Check sheet for the modelled part. Datum: model origin and axes. Units: mm. A direction names the side the tool comes from. Coordinates: 2 decimals unless noted, no trailing zeros. Loops run counter-clockwise (first coordinate to the right, second up) from the corner with the lowest first, then second, coordinate; pieces in that order, holes last. Notation, with made-up numbers: (73, 16) -> (90, 16) arc R16 ccw to (90, 25) -> close; hole circle Ø3 at (-1.75, 37). An arc over 180 degrees is marked (long way). Use one line per item in the form item = value.
from build123d import *

# Parameters (mm, degrees)
SKETCH2_R           = 3
BOSS_EXTRUDE1_DEPTH = 1


with BuildPart() as part:
    # Sketch1 → Revolve1 (revolve)
    with BuildSketch(Plane.XY, mode=Mode.PRIVATE) as revolve1_sk:
        Polygon((0, 0), (2.5, 0), (2.5, 4), (7.5, 4), (7.5, 6), (10, 6), (10, 4), (12.497669608, 4), (12.497669608, 14), (10, 14), (10, 12), (7.5, 12), (7.5, 14), (5, 14), (5, 29), (0, 29), align=None)
    revolve(revolve1_sk.sketch.rotate(Axis((0, 0, 0), (0, 1, 0)), 90), axis=Axis((0, 0, 0), (0, 1, 0)))

    # Sketch2 → Boss-Extrude1 (add)
    with BuildSketch(Plane.XZ.offset(-4)):
        with Locations(Location((0, 0, 0), (0, 0, 270))):
            Circle(SKETCH2_R)
    extrude(amount=BOSS_EXTRUDE1_DEPTH)


solid = part.part
(1) Section check C-C, the plane z = 6.25. Record the boundary of the cut face in (x, y).
Established:
outline = (-10.82, 4) -> (-7.81, 4) -> (-7.81, 6) -> (-4.15, 6) -> (-4.15, 4) -> (4.15, 4) -> (4.15, 6) -> (7.81, 6) -> (7.81, 4) -> (10.82, 4) -> (10.82, 14) -> (7.81, 14) -> (7.81, 12) -> (4.15, 12) -> (4.15, 14) -> (-4.15, 14) -> (-4.15, 12) -> (-7.81, 12) -> (-7.81, 14) -> (-10.82, 14) -> close
(2) Scan lines: line 1 along X through (y, z) = (5.45, 0); line 2 along Y through (x, z) = (-10.75, 0.75); line 3 along Y through (x, z) = (8.75, 3). Record each from-to range of solid material in increasing order.
Established:
line_1 = -12.5 to -10, -7.5 to 7.5, 10 to 12.5
line_2 = 4 to 14
line_3 = 6 to 12
(3) Mould release check, pull along X, two halves, no side actions. Record for faces 4 (the cylindrical face through (0, 5, 10)), 5 (the flat face through (0, 29, 0)), 6 (the cylindrical face through (0.9, 3.51, -2.86)): +X half, -X half, draft (parallel to the pull), parting line (faces both ways), or undercut.
Established:
face_4 = undercut
face_5 = draft
face_6 = parting line
(4) Tool access check on faces 1 (the flat face through (0, 0, 0)), 2 (the cylindrical face through (-6.324, 13.014, -4.032)), 3 (the flat face through (-7, 6, 4)). Record the directions out of +Z, -Z, +X, -X, +Y, -Y that give a thin tool (end or side, any length) a straight path to the whole face; none if there is none.
Established:
face_1 = +Z, -Z, +X, -X, -Y
face_2 = +Y
face_3 = -Y
(5) Section check D-D, the plane x = -9. Record the boundary of the cut face in (y, z), plus the area to 3 significant figures.
Established:
outline = (4, -8.67) -> (14, -8.67) -> (14, -4.36) -> (12, -4.36) -> (12, 4.36) -> (14, 4.36) -> (14, 8.67) -> (4, 8.67) -> (4, 4.36) -> (6, 4.36) -> (6, -4.36) -> (4, -4.36) -> close
area = 139 mm²
(6) Go/stop test with flat-tipped pins: P1, Ø5, axis at y = 3.5, z = -4, coming from the -X side; P2, Ø6, axis at x = -2, y = 24.5, coming from the -Z side; P3, Ø3, axis at x = -8.5, z = -6.5, coming from the -Y side. Record where each tip stops, or that it passes through.
Established:
P1 = -12.4
P2 = -5
P3 = 4
